```python
from build123d import *

# Parameters (mm, degrees)
SKIZZE1_W                       = 57
SKIZZE1_H                       = 57
AUFSATZ_LINEAR_AUSTRAGEN1_DEPTH = 150
SKIZZE2_R                       = 19.05
AUFSATZ_LINEAR_AUSTRAGEN2_DEPTH = 2
AUFSATZ_LINEAR_AUSTRAGEN3_DEPTH = 21
SKIZZE4_R                       = 2.7
SCHNITT_LINEAR_AUSTRAGEN1_DEPTH = 50
SCHNITT_LINEAR_START            = -7
SCHNITT_LINEAR_AUSTRAGEN2_DEPTH = 170
SKIZZE6_W                       = 80
SKIZZE6_H                       = 52
AUFSATZ_LINEAR_AUSTRAGEN4_DEPTH = 16
VERRUNDUNG1_R                   = 10
SKIZZE7_W                       = 10.157968888
SKIZZE7_H                       = 35.311034703
SKIZZE7_W_2                     = 8.384355272
AUFSATZ_LINEAR_AUSTRAGEN5_DEPTH = 16


with BuildPart() as part:
    # Skizze1 → Aufsatz-Linear austragen1 (new body)
    with BuildSketch(Plane.XY):
        Rectangle(SKIZZE1_W, SKIZZE1_H)
    extrude(amount=AUFSATZ_LINEAR_AUSTRAGEN1_DEPTH)

    # Skizze2 → Aufsatz-Linear austragen2 (add)
    with BuildSketch(Plane(origin=(0, 0, 0), x_dir=(-1, 0, 0), z_dir=(0, 0, -1))):
        with Locations(Location((0, 0, 0), (0, 0, 180))):
            Circle(SKIZZE2_R)
    extrude(amount=AUFSATZ_LINEAR_AUSTRAGEN2_DEPTH)

    # Skizze3 → Aufsatz-Linear austragen3 (add)
    with BuildSketch(Plane(origin=(0, 0, -2), x_dir=(-1, 0, 0), z_dir=(0, 0, -1))):
        with BuildLine():
            Line((-1.936491673, -3.5), (1.936491673, -3.5))
            ThreePointArc((1.936491673, -3.5), (0, 4), (-1.936491673, -3.5))
        make_face()
    extrude(amount=AUFSATZ_LINEAR_AUSTRAGEN3_DEPTH)

    # Skizze4 → Schnitt-Linear austragen1 (cut)
    with BuildSketch(Plane(origin=(0, 0, 0), x_dir=(-1, 0, 0), z_dir=(0, 0, -1))):
        with Locations((23.55, 23.55)):
            Circle(SKIZZE4_R)
        with Locations(Location((-23.55, 23.55, 0), (0, 0, 180))):
            Circle(SKIZZE4_R)
        with Locations(Location((23.55, -23.55, 0), (0, 0, 180))):
            Circle(SKIZZE4_R)
        with Locations((-23.55, -23.55)):
            Circle(SKIZZE4_R)
    extrude(amount=-SCHNITT_LINEAR_AUSTRAGEN1_DEPTH, mode=Mode.SUBTRACT)

    # Skizze5 → Schnitt-Linear austragen2 (cut)
    with BuildSketch(Plane(origin=(0, 0, 0), x_dir=(-1, 0, 0), z_dir=(0, 0, -1)).offset(SCHNITT_LINEAR_START)):
        with BuildLine():
            Line((18.5, 23.55), (18.5, 28.5))
            Line((18.5, 28.5), (28.5, 28.5))
            Line((28.5, 28.5), (28.5, 18.5))
            Line((28.5, 18.5), (23.55, 18.5))
            ThreePointArc((23.55, 18.5), (19.979110755, 19.979110755), (18.5, 23.55))
        make_face()
        with BuildLine():
            Line((-28.5, 28.5), (-28.5, 18.5))
            Line((-28.5, 18.5), (-23.55, 18.5))
            ThreePointArc((-23.55, 18.5), (-19.979110755, 19.979110755), (-18.5, 23.55))
            Line((-18.5, 23.55), (-18.5, 28.5))
            Line((-18.5, 28.5), (-28.5, 28.5))
        make_face()
        with BuildLine():
            Line((28.5, -18.5), (23.55, -18.5))
            ThreePointArc((23.55, -18.5), (19.979110755, -19.979110755), (18.5, -23.55))
            Line((18.5, -23.55), (18.5, -28.5))
            Line((18.5, -28.5), (28.5, -28.5))
            Line((28.5, -28.5), (28.5, -18.5))
        make_face()
        with BuildLine():
            Line((-28.5, -18.5), (-23.55, -18.5))
            ThreePointArc((-23.55, -18.5), (-19.979110755, -19.979110755), (-18.5, -23.55))
            Line((-18.5, -23.55), (-18.5, -28.5))
            Line((-18.5, -28.5), (-28.5, -28.5))
            Line((-28.5, -28.5), (-28.5, -18.5))
        make_face()
    extrude(amount=-SCHNITT_LINEAR_AUSTRAGEN2_DEPTH, mode=Mode.SUBTRACT)

    # Skizze6 → Aufsatz-Linear austragen4 (add)
    with BuildSketch(Plane.ZY.offset(28.5)):
        with Locations((108, 0)):
            Rectangle(SKIZZE6_W, SKIZZE6_H)
    extrude(amount=AUFSATZ_LINEAR_AUSTRAGEN4_DEPTH)

    # Verrundung1
    # the kernel refuses this fillet: 10 mm, written as the material it takes off along each edge
    with BuildSketch(Plane(origin=(-28.5, 26, 68), x_dir=(0, -1, 0), z_dir=(-1, 0, 0))) as verrundung1_piece_1:
        with BuildLine():
            CenterArc((VERRUNDUNG1_R, VERRUNDUNG1_R), VERRUNDUNG1_R, 180, 90)
            Line((0, VERRUNDUNG1_R), (0, 0))
            Line((0, 0), (VERRUNDUNG1_R, 0))
        make_face()
    extrude(amount=41, mode=Mode.SUBTRACT)
    with BuildSketch(Plane(origin=(-28.5, -26, 68), x_dir=(0, 1, 0), z_dir=(-1, 0, 0))) as verrundung1_piece_2:
        with BuildLine():
            CenterArc((VERRUNDUNG1_R, -VERRUNDUNG1_R), VERRUNDUNG1_R, 90, 90)
            Line((0, -VERRUNDUNG1_R), (0, 0))
            Line((0, 0), (VERRUNDUNG1_R, 0))
        make_face()
    extrude(amount=41, mode=Mode.SUBTRACT)

    # Skizze7 → Aufsatz-Linear austragen5 (add)
    with BuildSketch(Plane.ZY.offset(44.5)):
        with Locations((88.733684617, -0.161237601)):
            Rectangle(SKIZZE7_W, SKIZZE7_H)
        with Locations((115.579745248, -0.161237601)):
            Rectangle(SKIZZE7_W_2, SKIZZE7_H)
    extrude(amount=AUFSATZ_LINEAR_AUSTRAGEN5_DEPTH)


solid = part.part
```
The listing builds one solid part. Answer for the finished solid, in the listing's coordinates (mm). A direction names the side the tool comes from. Coordinates: 2 decimals unless noted, no trailing zeros. Write each loop counter-clockwise with the first axis right and the second up, starting at its lowest first coordinate (ties: lowest second). Pieces come first, ordered by that corner, then holes. Notation, with made-up numbers: (-23.5, -20) - (-17.5, -20) arc R10 ccw to (-17.5, -16) - close; hole circle Ø4 at (63, 69). An arc over 180 degrees is marked (long way). Return JSON: item names as keys, results as strings. Group by question number.
Q1. For a pull along X with two mould halves and no side action, classify faces 1 (the flat face through (-28.5, 0, 34)), 2 (the flat face through (-52, 0, 93.813)), 3 (the cylindrical face through (-22.965, 20.914, 3.451)) as +X half, -X half, draft (parallel to the pull), parting line (faces both ways), or undercut.
Q2. Find the intervals of material crossed by line 1 along Y through (x, z) = (23.55, 2.75); line 2 along Z through (x, y) = (-50.5, 13.5); line 3 along X through (y, z) = (24, 96), in increasing order. Write a range as [from, to].
Q3. The part is cut by section D-D on z = 72. Write down the section's boundary in (x, y).
Q4. The part is cut by section C-C on y = 0. Write down the section's boundary in (x, z).
Q5. The part is cut by section A-A on x = 0. Write down the section's boundary in (y, z).
Q6. The part is cut by section B-B on z = 42. Write down the section's boundary in (x, y).
Q7. Which of the six approach directions +Z, -Z, +X, -X, +Y, -Y give full straight-line access (tool end or side, diameter ignored) to faces 4 (the flat face through (26, -26, 7)), 5 (the cylindrical face through (-36.39, 23.15, 71.01)), 6 (the flat face through (-52, 0, 119.772)), 7 (the flat face through (-36, 26, 113))?
Q8. Flat-ended cylindrical pins translate along their axes: pin 1 Ø5 at (x, y) = (-55, 6) entering from +Z; pin 2 Ø8 at (x, y) = (23, 22.5) entering from +Z; pin 3 Ø7 at (x, y) = (-23.55, -23.55) entering from -Z; pin 4 Ø1.9 at (x, z) = (-0.5, -11.5) entering from -Y. Find the tip coordinate at first contact, or state that the pin passes through.
Evaluation:
{
 "1": {"face 1": "-X half", "face 2": "draft", "face 3": "undercut"},
 "2": {"line 1": "y = [-28.5, -26.25], [-20.85, 20.85], [26.25, 28.5]", "line 2": "z = [83.65, 93.81], [111.39, 119.77]", "line 3": "x = [-44.5, -28.5], [-18.5, 18.5]"},
 "3": {"outline": "(-44.5, -24) - (-28.5, -24) - (-28.5, -18.5) - (-23.55, -18.5) arc R5.05 cw to (-18.5, -23.55) - (-18.5, -28.5) - (18.5, -28.5) - (18.5, -23.55) arc R5.05 cw to (23.55, -18.5) - (28.5, -18.5) - (28.5, 18.5) - (23.55, 18.5) arc R5.05 cw to (18.5, 23.55) - (18.5, 28.5) - (-18.5, 28.5) - (-18.5, 23.55) arc R5.05 cw to (-23.55, 18.5) - (-28.5, 18.5) - (-28.5, 24) - (-44.5, 24) - close"},
 "4": {"outline": "(-60.5, 83.65) - (-44.5, 83.65) - (-44.5, 68) - (-28.5, 68) - (-28.5, 0) - (-19.05, 0) - (-19.05, -2) - (-4, -2) - (-4, -23) - (4, -23) - (4, -2) - (19.05, -2) - (19.05, 0) - (28.5, 0) - (28.5, 150) - (-28.5, 150) - (-28.5, 148) - (-44.5, 148) - (-44.5, 119.77) - (-60.5, 119.77) - (-60.5, 111.39) - (-44.5, 111.39) - (-44.5, 93.81) - (-60.5, 93.81) - close"},
 "5": {"outline": "(-28.5, 0) - (-19.05, 0) - (-19.05, -2) - (-3.5, -2) - (-3.5, -23) - (4, -23) - (4, -2) - (19.05, -2) - (19.05, 0) - (28.5, 0) - (28.5, 150) - (-28.5, 150) - close"},
 "6": {"outline": "(-28.5, -18.5) - (-23.55, -18.5) arc R5.05 cw to (-18.5, -23.55) - (-18.5, -28.5) - (18.5, -28.5) - (18.5, -23.55) arc R5.05 cw to (23.55, -18.5) - (28.5, -18.5) - (28.5, 18.5) - (23.55, 18.5) arc R5.05 cw to (18.5, 23.55) - (18.5, 28.5) - (-18.5, 28.5) - (-18.5, 23.55) arc R5.05 cw to (-23.55, 18.5) - (-28.5, 18.5) - close"},
 "7": {"face 4": "+Z, +X, -Y", "face 5": "-Z, -X, +Y", "face 6": "+Z, -X, +Y, -Y", "face 7": "+Z, -Z, -X, +Y"},
 "8": {"pin 1": "stops at z = 119.77", "pin 2": "stops at z = 150", "pin 3": "stops at z = 0", "pin 4": "stops at y = -3.5"}
}
